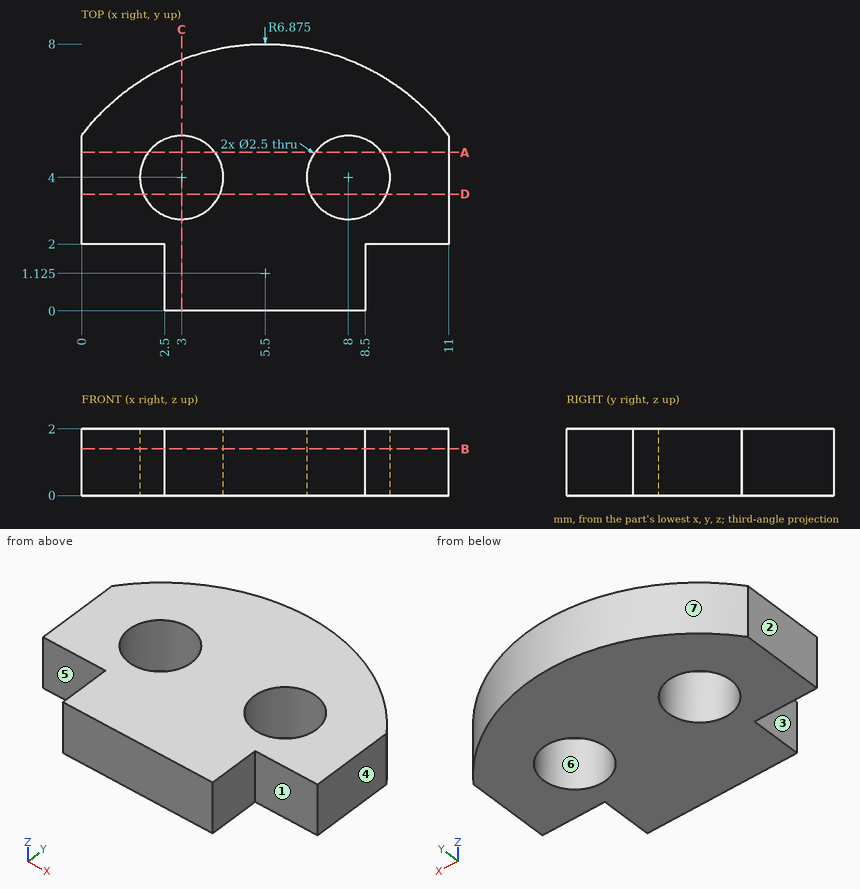
Design review of the part shown in the three views and the two pictorial views. Dimensions are in mm from the part's minimum x, y and z. A direction names the side the tool comes from. Round coordinates to 2 decimals unless told otherwise and drop trailing zeros. Write each loop counter-clockwise with the first axis right and the second up, starting at its lowest first coordinate (ties: lowest second). Pieces come first, ordered by that corner, then holes.
Item 1: We need section B-B on z = 1.4. Write out the cut boundary in (x, y) (3 decimals), and give its area (3 significant figures).
Item 2: Clearance check with flat-ended pins moving along their axes: pin 1 Ø0.6 at (y, z) = (1, 1.5) entering from -X; pin 2 Ø0.6 at (x, z) = (10, 1) entering from -Y. State where each tip first meets the part, or that it passes through.
Item 3: For the marked faces 1, 2 and 3, list the 3-axis set-ups (+Z, -Z, +X, -X, +Y, -Y) from which the entire face can be reached by the end or side of a thin tool; tool diameter is ignored.
Item 4: We need section A-A on y = 4.75. Write out the cut boundary in (x, z), and give its area (3 significant figures).
Item 5: The part is to be moulded in two halves that separate along Y. For the marked faces 4, 5, 6 and 7, say which applies: +Y half, -Y half, draft (parallel to the pull), parting line (faces both ways), or undercut.
Item 6: We need section C-C on x = 3. Write out the cut boundary in (y, z).
Item 7: For probe 1 along X at (y, z) = (4, 0.9); probe 2 along X at (y, z) = (4.75, 0.6); probe 3 along Y at (x, z) = (7.5, 1.7), list the stretches that pass through material, from the lowest coordinate up.
Item 8: We need section D-D on y = 3.5. Write out the cut boundary in (x, z).
Returned:
1. outline: (0, 2) - (2.5, 2) - (2.5, 0) - (8.5, 0) - (8.5, 2) - (11, 2) - (11, 5.25) arc R6.875 ccw to (0, 5.25) - close; hole circle Ø2.5 at (3, 4); hole circle Ø2.5 at (8, 4)
1. area: 59.1 mm2
2. pin 1: stops at x = 2.5
2. pin 2: stops at y = 2
3. face 1: +Z, -Z, +X, -Y
3. face 2: +Z, -Z, -X, +Y, -Y
3. face 3: +Z, -Z, -X, -Y
4. outline: (0, 0) - (2, 0) - (2, 2) - (0, 2) - close; (4, 0) - (7, 0) - (7, 2) - (4, 2) - close; (9, 0) - (11, 0) - (11, 2) - (9, 2) - close
4. area: 14.0 mm2
5. face 4: draft
5. face 5: -Y half
5. face 6: undercut
5. face 7: +Y half
6. outline: (0, 0) - (2.75, 0) - (2.75, 2) - (0, 2) - close; (5.25, 0) - (7.53, 0) - (7.53, 2) - (5.25, 2) - close
7. probe 1: x = 0 to 1.75, 4.25 to 6.75, 9.25 to 11
7. probe 2: x = 0 to 2, 4 to 7, 9 to 11
7. probe 3: y = 0 to 2.85, 5.15 to 7.7
8. outline: (0, 0) - (1.85, 0) - (1.85, 2) - (0, 2) - close; (4.15, 0) - (6.85, 0) - (6.85, 2) - (4.15, 2) - close; (9.15, 0) - (11, 0) - (11, 2) - (9.15, 2) - close
